Geometry: final body of the model. Coordinates: model frame, mm. Face numbers are marked on the shaded views. A direction names the side the tool comes from. Give positions to 0.01 mm unless a question says otherwise; leave off trailing zeros. Write each loop counter-clockwise with the first axis right and the second up, starting at its lowest first coordinate (ties: lowest second). Pieces come first, ordered by that corner, then holes.
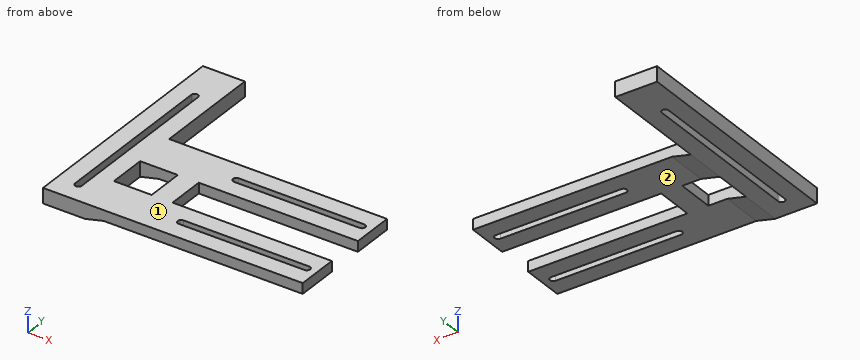
```python
from build123d import *

# Parameters (mm, degrees)
SKETCH_1_W                  = 76
SKETCH_1_H                  = 20
SKETCH_1_W_2                = 18
SKETCH_1_W_3                = 10
SKETCH_1_H_2                = 18
SKETCH_1_W_4                = 20
SKETCH_1_H_3                = 52.041621827
EXTRUDE_1_DEPTH             = 5
HOLE_WIZARD_3_2_3_2_1_DEPTH = 5
SKETCH_8_W                  = 20
SKETCH_8_H                  = 110.041621827
EXTRUDE_2_DEPTH             = 2.2
HOLE_START                  = -2.2
HOLE_WIZARD_3_2_3_2_3_DEPTH = 7.2
RIB_1_REACH                 = 147.55
SKETCH_11_WALL_W            = 302.364540162
SKETCH_11_WALL_H            = 20
RIB_2_REACH                 = 113.533
SKETCH_12_WALL_W            = 234.330707354
SKETCH_12_WALL_H            = 20


# Read off the part's stored shape, not the designer's step: Ø3.2 (3.2) 直径槽口1, Ø3.2 (3.2) 直径槽口3
with BuildPart() as part:
    # 草图1 → 凸台-拉伸1 (new body)
    with BuildSketch(Plane.XY):
        with Locations((-9.134530028, -25.635533007)):
            Rectangle(SKETCH_1_W, SKETCH_1_H)
        with Locations((-66.134530028, -25.635533007)):
            Rectangle(SKETCH_1_W_2, SKETCH_1_H)
        with Locations((-52.134530028, -25.635533007)):
            Rectangle(SKETCH_1_W_3, SKETCH_1_H)
        with Locations((-66.134530028, 12.364466993)):
            Rectangle(SKETCH_1_W_2, SKETCH_1_H)
        with Locations((-9.134530028, 12.364466993)):
            Rectangle(SKETCH_1_W, SKETCH_1_H)
        with Locations((-52.134530028, 12.364466993)):
            Rectangle(SKETCH_1_W_3, SKETCH_1_H)
        with Locations((-52.134530028, -6.635533007)):
            Rectangle(SKETCH_1_W_3, SKETCH_1_H_2)
        with Locations((-85.134530028, 12.364466993)):
            Rectangle(SKETCH_1_W_4, SKETCH_1_H)
        with Locations((-85.134530028, -6.635533007)):
            Rectangle(SKETCH_1_W_4, SKETCH_1_H_2)
        with Locations((-85.134530028, -25.635533007)):
            Rectangle(SKETCH_1_W_4, SKETCH_1_H)
        with Locations((-85.134530028, 48.385277907)):
            Rectangle(SKETCH_1_W_4, SKETCH_1_H_3)
    extrude(amount=EXTRUDE_1_DEPTH)

    # Ø3.2 (3.2) 直径槽口1 outline → Ø3.2 (3.2) 直径槽口1 (cut)
    with BuildSketch(Plane.XY):
        with BuildLine():
            Line((-36.134530028, 10.764466993), (23.865469972, 10.764466993))
            ThreePointArc((23.865469972, 10.764466993), (25.465469972, 12.364466993), (23.865469972, 13.964466993))
            Line((23.865469972, 13.964466993), (-36.134530028, 13.964466993))
            ThreePointArc((-36.134530028, 13.964466993), (-37.734530028, 12.364466993), (-36.134530028, 10.764466993))
        make_face()
        with BuildLine():
            Line((-36.134530028, -27.235533007), (23.865469972, -27.235533007))
            ThreePointArc((23.865469972, -27.235533007), (25.465469972, -25.635533007), (23.865469972, -24.035533007))
            Line((23.865469972, -24.035533007), (-36.134530028, -24.035533007))
            ThreePointArc((-36.134530028, -24.035533007), (-37.734530028, -25.635533007), (-36.134530028, -27.235533007))
        make_face()
    extrude(amount=HOLE_WIZARD_3_2_3_2_1_DEPTH, mode=Mode.SUBTRACT)

    # 草图8 → 凸台-拉伸2 (add)
    with BuildSketch(Plane(origin=(0, 0, 0), x_dir=(-1, 0, 0), z_dir=(0, 0, -1))):
        with Locations((85.134530028, 19.385277907)):
            Rectangle(SKETCH_8_W, SKETCH_8_H)
    extrude(amount=EXTRUDE_2_DEPTH)

    # Ø3.2 (3.2) 直径槽口3 outline → Ø3.2 (3.2) 直径槽口3 (cut)
    with BuildSketch(Plane.XY.offset(HOLE_START)):
        with BuildLine():
            Line((-83.534530028, -25.635533007), (-83.534530028, 54.364466993))
            ThreePointArc((-83.534530028, 54.364466993), (-85.134530028, 55.964466993), (-86.734530028, 54.364466993))
            Line((-86.734530028, 54.364466993), (-86.734530028, -25.635533007))
            ThreePointArc((-86.734530028, -25.635533007), (-85.134530028, -27.235533007), (-83.534530028, -25.635533007))
        make_face()
    extrude(amount=HOLE_WIZARD_3_2_3_2_3_DEPTH, mode=Mode.SUBTRACT)

    # 草图11 wall → 筋1 (add, up to next)
    with BuildSketch(Plane(origin=(-70.634530028, -35.635533007, -1.1), x_dir=(0.971399006497, 0, 0.237453090477), z_dir=(-0.237453090477, 0, 0.971399006497)), mode=Mode.PRIVATE) as rib_1_sk1:
        with Locations((0, 10)):
            Rectangle(SKETCH_11_WALL_W, SKETCH_11_WALL_H)
    rib_1_tool1 = extrude(rib_1_sk1.sketch, amount=RIB_1_REACH, mode=Mode.PRIVATE) - part.part
    add(rib_1_tool1.solids().sort_by_distance((-70.634530028, -35.635533007, -1.1))[0])

    # 草图12 wall → 筋2 (add, up to next)
    with BuildSketch(Plane(origin=(-70.634530028, 22.364466993, -1.1), x_dir=(0.971399006497, 0, 0.237453090477), z_dir=(0.237453090477, 0, -0.971399006497)), mode=Mode.PRIVATE) as rib_2_sk1:
        with Locations((0, 10)):
            Rectangle(SKETCH_12_WALL_W, SKETCH_12_WALL_H)
    rib_2_tool1 = extrude(rib_2_sk1.sketch, amount=-RIB_2_REACH, mode=Mode.PRIVATE) - part.part
    add(rib_2_tool1.solids().sort_by_distance((-70.634530028, 22.364466993, -1.1))[0])


solid = part.part
```
Item 1: Section D-D, the plane z = 3.25. Return the cut outline in (x, y), plus the area to 3 significant figures.
Found:
outline: (-95.13, -35.64) - (28.87, -35.64) - (28.87, -15.64) - (-47.13, -15.64) - (-47.13, 2.36) - (28.87, 2.36) - (28.87, 22.36) - (-75.13, 22.36) - (-75.13, 74.41) - (-95.13, 74.41) - close; hole (-86.73, -25.64) arc R1.6 ccw to (-83.53, -25.64) - (-83.53, 54.36) arc R1.6 ccw to (-86.73, 54.36) - close; hole (-75.13, -15.64) - (-57.13, -15.64) - (-57.13, 2.36) - (-75.13, 2.36) - close; hole (-36.13, -27.24) - (23.87, -27.24) arc R1.6 ccw to (23.87, -24.04) - (-36.13, -24.04) arc R1.6 ccw to start; hole (-36.13, 10.76) - (23.87, 10.76) arc R1.6 ccw to (23.87, 13.96) - (-36.13, 13.96) arc R1.6 ccw to start
area: 5,880 mm2
Item 2: Section A-A, the plane y = -21. Return the cut outline in (x, z), plus the area to 3 significant figures.
Found:
outline: (-95.13, -2.2) - (-86.73, -2.2) - (-86.73, 5) - (-95.13, 5) - close; (-83.53, -2.2) - (-75.13, -2.2) - (-66.13, 0) - (28.87, 0) - (28.87, 5) - (-83.53, 5) - close
area: 651 mm2
Item 3: Section B-B, the plane x = -59.5. Return the cut outline in (y, z), plus the area to 3 significant figures.
Found:
outline: (-35.64, 0) - (-15.64, 0) - (-15.64, 5) - (-35.64, 5) - close; (2.36, 0) - (22.36, 0) - (22.36, 5) - (2.36, 5) - close
area: 200 mm2
Item 4: Section C-C, the plane x = -28. Return the cut outline in (y, z).
Found:
outline: (-35.64, 0) - (-27.24, 0) - (-27.24, 5) - (-35.64, 5) - close; (-24.04, 0) - (-15.64, 0) - (-15.64, 5) - (-24.04, 5) - close; (2.36, 0) - (10.76, 0) - (10.76, 5) - (2.36, 5) - close; (13.96, 0) - (22.36, 0) - (22.36, 5) - (13.96, 5) - close
Item 5: Reachability of the marked faces 1 and 2 from +Z, -Z, +X, -X, +Y, -Y: full face, straight path, thin tool, end or side. Return the list, or none.
Found:
face 1: +Z, +X, -X, +Y, -Y
face 2: -Z, +X, +Y, -Y
Item 6: Line query: L1, parallel to X at y = -4, z = 0.5; L2, parallel to X at y = -25.5, z = 3.75; L3, parallel to Y at x = 9, z = 2.25. Output: solid intervals per line, ascending.
Found:
L1: x = -95.13 to -86.73, -83.53 to -75.13, -57.13 to -47.13
L2: x = -95.13 to -86.73, -83.53 to -37.73, 25.46 to 28.87
L3: y = -35.64 to -27.24, -24.04 to -15.64, 2.36 to 10.76, 13.96 to 22.36
Item 7: Pin query (flat end, axial travel): pin 1 Ø2 at (x, z) = (-73.5, 1.5) entering from +Y; pin 2 Ø1.5 at (y, z) = (-3.5, 3.5) entering from +X. Return the tip coordinate at first contact, or that it passes through.
Found:
pin 1: stops at y = 22.36
pin 2: stops at x = -47.13
